```python
from build123d import *

# Parameters (mm, degrees)
F1_DEPTH = 5.6
F2_DEPTH = 7
F0_W     = 75.5
F0_H     = 51
F3_DEPTH = 2
F4_R     = 1.99999
F5_SIZE2 = 1.99999
F5_SIZE  = 2.99999
F6_R     = 1.25
F7_DEPTH = 5


# Not quite as in the source:
# - a fillet or chamfer is up to 0.001 mm smaller than in the source, because OpenCascade refuses the exact size


with BuildPart() as f1:
    # F0 (on Top) → F1 (new body)
    with BuildSketch(Plane.XY):
        with BuildLine():
            ThreePointArc((-34.4414402544, 28.4581715763), (-31.2414402544, 25.2581715763), (-28.0414402544, 28.4581715763))
            ThreePointArc((-28.0414402544, 28.4581715763), (-28.9786985547, 30.7209132761), (-31.2414402544, 31.6581715763))
            ThreePointArc((-31.2414402544, 31.6581715763), (-33.5041819542, 30.7209132761), (-34.4414402544, 28.4581715763))
        make_face()
    extrude(amount=F1_DEPTH)



with BuildPart() as f1b:
    # F0 (on Top) → F1, piece 2 (new body)
    with BuildSketch(Plane.XY):
        with BuildLine():
            ThreePointArc((-28.0414402544, -20.0818284237), (-31.2414402544, -16.8818284237), (-34.4414402544, -20.0818284237))
            ThreePointArc((-34.4414402544, -20.0818284237), (-33.5041819542, -22.3445701235), (-31.2414402544, -23.2818284237))
            ThreePointArc((-31.2414402544, -23.2818284237), (-28.9786985547, -22.3445701235), (-28.0414402544, -20.0818284237))
        make_face()
    extrude(amount=F1_DEPTH)


with BuildPart() as f1c:
    # F0 (on Top) → F1, piece 3 (new body)
    with BuildSketch(Plane.XY):
        with BuildLine():
            ThreePointArc((62.8585597456, -23.2818284237), (65.1213014453, -22.3445701235), (66.0585597456, -20.0818284237))
            ThreePointArc((66.0585597456, -20.0818284237), (60.5958180458, -17.8190867239), (62.8585597456, -23.2818284237))
        make_face()
    extrude(amount=F1_DEPTH)


with BuildPart() as f1d:
    # F0 (on Top) → F1, piece 4 (new body)
    with BuildSketch(Plane.XY):
        with BuildLine():
            ThreePointArc((66.0585597456, 28.4581715763), (65.1213014453, 30.7209132761), (62.8585597456, 31.6581715763))
            ThreePointArc((62.8585597456, 31.6581715763), (60.5958180458, 26.1954298765), (66.0585597456, 28.4581715763))
        make_face()
    extrude(amount=F1_DEPTH)


with BuildPart() as f2:
    # F0 (on Top) → F2 (new body)
    with BuildSketch(Plane.XY):
        with BuildLine():
            Line((65.8985597456, 34.4581715763), (-29.4414402544, 34.4581715763))
            ThreePointArc((-29.4414402544, 34.4581715763), (-34.9568731477, 32.1736044695), (-37.2414402544, 26.6581715763))
            Line((-37.2414402544, 26.6581715763), (-37.2414402544, -18.2818284237))
            ThreePointArc((-37.2414402544, -18.2818284237), (-34.9568731477, -23.797261317), (-29.4414402544, -26.0818284237))
            Line((-29.4414402544, -26.0818284237), (65.8985597456, -26.0818284237))
            ThreePointArc((65.8985597456, -26.0818284237), (71.4139926388, -23.797261317), (73.6985597456, -18.2818284237))
            Line((73.6985597456, -18.2818284237), (73.6985597456, 26.6581715763))
            ThreePointArc((73.6985597456, 26.6581715763), (71.4139926388, 32.1736044695), (65.8985597456, 34.4581715763))
        make_face()
        with BuildLine():
            ThreePointArc((62.8585597456, 32.8581709981), (65.9698291739, 31.5694410047), (67.2585591674, 28.4581715763))
            Line((67.2585591674, 28.4581715763), (67.2585591674, -20.0818284237))
            ThreePointArc((67.2585591674, -20.0818284237), (65.9698291739, -23.1930978521), (62.8585597456, -24.4818278456))
            Line((62.8585597456, -24.4818278456), (-31.2414402544, -24.4818278456))
            ThreePointArc((-31.2414402544, -24.4818278456), (-34.3527096828, -23.1930978521), (-35.6414396763, -20.0818284237))
            Line((-35.6414396763, -20.0818284237), (-35.6414396763, 28.4581715763))
            ThreePointArc((-35.6414396763, 28.4581715763), (-34.3527096828, 31.5694410047), (-31.2414402544, 32.8581709981))
            Line((-31.2414402544, 32.8581709981), (62.8585597456, 32.8581709981))
        make_face(mode=Mode.SUBTRACT)
    extrude(amount=F2_DEPTH)


with BuildPart() as f1_1:
    add(f1.part)

    add(f1b.part)  # F3 merges F1b

    add(f1c.part)  # F3 merges F1c

    add(f1d.part)  # F3 merges F1d

    add(f2.part)  # F3 merges F2
    # F0 (on Top) → F3 (join)
    with BuildSketch(Plane.XY):
        with BuildLine():
            Line((65.8985597456, 36.6581715763), (-29.4414402544, 36.6581715763))
            ThreePointArc((-29.4414402544, 36.6581715763), (-36.5125080663, 33.7292393881), (-39.4414402544, 26.6581715763))
            Line((-39.4414402544, 26.6581715763), (-39.4414402544, -18.2818284237))
            ThreePointArc((-39.4414402544, -18.2818284237), (-36.5125080663, -25.3528962356), (-29.4414402544, -28.2818284237))
            Line((-29.4414402544, -28.2818284237), (65.8985597456, -28.2818284237))
            ThreePointArc((65.8985597456, -28.2818284237), (72.9696275574, -25.3528962356), (75.8985597456, -18.2818284237))
            Line((75.8985597456, -18.2818284237), (75.8985597456, 26.6581715763))
            ThreePointArc((75.8985597456, 26.6581715763), (72.9696275574, 33.7292393881), (65.8985597456, 36.6581715763))
        make_face()
        with BuildLine():
            ThreePointArc((-37.2414402544, 26.6581715763), (-34.9568731477, 32.1736044695), (-29.4414402544, 34.4581715763))
            Line((-29.4414402544, 34.4581715763), (65.8985597456, 34.4581715763))
            ThreePointArc((65.8985597456, 34.4581715763), (71.4139926388, 32.1736044695), (73.6985597456, 26.6581715763))
            Line((73.6985597456, 26.6581715763), (73.6985597456, -18.2818284237))
            ThreePointArc((73.6985597456, -18.2818284237), (71.4139926388, -23.797261317), (65.8985597456, -26.0818284237))
            Line((65.8985597456, -26.0818284237), (-29.4414402544, -26.0818284237))
            ThreePointArc((-29.4414402544, -26.0818284237), (-34.9568731477, -23.797261317), (-37.2414402544, -18.2818284237))
            Line((-37.2414402544, -18.2818284237), (-37.2414402544, 26.6581715763))
        make_face(mode=Mode.SUBTRACT)
        with BuildLine():
            Line((67.2585591674, -20.0818284237), (67.2585591674, 28.4581715763))
            ThreePointArc((67.2585591674, 28.4581715763), (65.9698291739, 31.5694410047), (62.8585597456, 32.8581709981))
            Line((62.8585597456, 32.8581709981), (-31.2414402544, 32.8581709981))
            ThreePointArc((-31.2414402544, 32.8581709981), (-34.3527096828, 31.5694410047), (-35.6414396763, 28.4581715763))
            Line((-35.6414396763, 28.4581715763), (-35.6414396763, -20.0818284237))
            ThreePointArc((-35.6414396763, -20.0818284237), (-34.3527096828, -23.1930978521), (-31.2414402544, -24.4818278456))
            Line((-31.2414402544, -24.4818278456), (62.8585597456, -24.4818278456))
            ThreePointArc((62.8585597456, -24.4818278456), (65.9698291739, -23.1930978521), (67.2585591674, -20.0818284237))
        make_face()
        with BuildLine():
            ThreePointArc((-34.4414402544, 28.4581715763), (-33.5041819542, 30.7209132761), (-31.2414402544, 31.6581715763))
            Line((-31.2414402544, 31.6581715763), (62.8585597456, 31.6581715763))
            ThreePointArc((62.8585597456, 31.6581715763), (65.1213014453, 30.7209132761), (66.0585597456, 28.4581715763))
            Line((66.0585597456, 28.4581715763), (66.0585597456, -20.0818284237))
            ThreePointArc((66.0585597456, -20.0818284237), (65.1213014453, -22.3445701235), (62.8585597456, -23.2818284237))
            Line((62.8585597456, -23.2818284237), (-31.2414402544, -23.2818284237))
            ThreePointArc((-31.2414402544, -23.2818284237), (-33.5041819542, -22.3445701235), (-34.4414402544, -20.0818284237))
            Line((-34.4414402544, -20.0818284237), (-34.4414402544, 28.4581715763))
        make_face(mode=Mode.SUBTRACT)
        with BuildLine():
            ThreePointArc((-31.2414402544, 31.6581715763), (-28.9786985547, 30.7209132761), (-28.0414402544, 28.4581715763))
            ThreePointArc((-28.0414402544, 28.4581715763), (-31.2414402544, 25.2581715763), (-34.4414402544, 28.4581715763))
            Line((-34.4414402544, 28.4581715763), (-34.4414402544, -20.0818284237))
            ThreePointArc((-34.4414402544, -20.0818284237), (-31.2414402544, -16.8818284237), (-28.0414402544, -20.0818284237))
            ThreePointArc((-28.0414402544, -20.0818284237), (-28.9786985547, -22.3445701235), (-31.2414402544, -23.2818284237))
            Line((-31.2414402544, -23.2818284237), (62.8585597456, -23.2818284237))
            ThreePointArc((62.8585597456, -23.2818284237), (60.5958180458, -17.8190867239), (66.0585597456, -20.0818284237))
            Line((66.0585597456, -20.0818284237), (66.0585597456, 28.4581715763))
            ThreePointArc((66.0585597456, 28.4581715763), (60.5958180458, 26.1954298765), (62.8585597456, 31.6581715763))
            Line((62.8585597456, 31.6581715763), (-31.2414402544, 31.6581715763))
        make_face()
        with Locations((18.2285597456, 4.1881715763)):
            Rectangle(F0_W, F0_H, mode=Mode.SUBTRACT)
    extrude(amount=F3_DEPTH)

    # F4 (radius 2 in the source; OpenCascade refuses exactly that, so slightly less here)
    f4_edges = [f1_1.edges().sort_by_distance(p)[0] for p in [
        (-36.512508, -25.352896, 0),
    ]]
    fillet(f4_edges, radius=F4_R)

    # F5 (size 3 and 2 in the source; OpenCascade refuses exactly that, so slightly less here)
    f5_edges = [f1_1.edges().sort_by_distance(p)[0] for p in [
        (18.22856, 29.688172, 0),
        (-19.52144, 4.188172, 0),
        (18.22856, -21.311828, 0),
        (55.97856, 4.188172, 0),
    ]]
    f5_side = f1_1.faces().sort_by_distance((-34.200797, -23.041185, 0))[0]
    chamfer(f5_edges, length=F5_SIZE, length2=F5_SIZE2, reference=f5_side)

    # F6 (on face) → F7 (cut)
    with BuildSketch(Plane.XY.offset(5.6)):
        with Locations((-31.2414402544, 28.4581715763)):
            Circle(F6_R)
        with Locations((-31.2414402544, -20.0818284237)):
            Circle(F6_R)
        with Locations((62.8585597456, -20.0818284237)):
            Circle(F6_R)
        with Locations((62.8585597456, 28.4581715763)):
            Circle(F6_R)
    extrude(amount=-F7_DEPTH, mode=Mode.SUBTRACT)


solid = f1_1.part
```
Input: part model. Units: mm. Frame: model coordinates. A direction names the side the tool comes from. Coordinates: 2 decimals unless noted, no trailing zeros. Return JSON: item names as keys, results as strings.
Q1. Ray query, probe 1 along X at (y, z) = (10, 3.25); probe 2 along Y at (x, z) = (59, 2.75); probe 3 along Z at (x, y) = (-31.5, 17). Return the intervals inside material, ascending.
The answers:
{"probe 1": "x = -37.24 to -35.64, 67.26 to 73.7", "probe 2": "y = -26.08 to -24.48, 32.86 to 34.46", "probe 3": "z = 0 to 2"}
Q2. Access query for faces 5 (the flat face through (-31, 28, 0.6)), 6 (the flat face through (-21, 3.789, 1.014)), 7 (the cylindrical face through (71.474, 32.113, 4.465)). Directions: +Z, -Z, +X, -X, +Y, -Y. A direction counts if a zero-diameter tool reaches every point of the face in a straight line with its end or side. Return the directions, or none.
The answers:
{"face 5": "+Z", "face 6": "-Z", "face 7": "+Z, +X, +Y"}
Q3. First-contact query: pin 1 (1.9 mm diameter, centred on x = -32.5, y = 27.5, fed in from +Z); pin 2 (3 mm diameter, centred on x = -20, z = 5, fed in from -Y); pin 3 (1.5 mm diameter, centred on x = 33.5, z = 5.5, fed in from +Y). Flat tips, straight axial feed; report the tip coordinate or a pass-through.
The answers:
{"pin 1": "stops at z = 5.6", "pin 2": "stops at y = -26.08", "pin 3": "stops at y = 34.46"}
Q4. Draft query along X for faces 1 (the flat face through (18, -26.082, 4)), 2 (the flat face through (57.46, 3.79, 1.01)), 3 (the cylindrical face through (75.297, 4.503, 0.57)), 4 (the cylindrical face through (-38.84, 3.87, 0.57)). Return one class per face: +X half, -X half, draft (parallel to the pull), parting line (faces both ways), or undercut.
The answers:
{"face 1": "draft", "face 2": "undercut", "face 3": "+X half", "face 4": "-X half"}
